```python
from build123d import *

# Parameters (mm, degrees)
ESQUISSE1_R                  = 53
ESQUISSE1_R_2                = 41
BOSS_EXTRU_1_DEPTH           = 3
ENL_V_MAT_EXTRU_1_DEPTH      = 76.013332148
ENL_V_MAT_EXTRU_1_DEPTH_BACK = 76.013332148
ENL_V_MAT_EXTRU_2_DEPTH      = 76.013332148
ENL_V_MAT_EXTRU_2_DEPTH_BACK = 76.013332148
CONG_1_R                     = 3
CONG_2_R                     = 2


with BuildPart() as part:
    # Esquisse1 → Boss.-Extru.1 (new body)
    with BuildSketch(Plane.XY):
        Circle(ESQUISSE1_R)
        Circle(ESQUISSE1_R_2, mode=Mode.SUBTRACT)
    extrude(amount=BOSS_EXTRU_1_DEPTH)

    # Esquisse2 → Enlèv. mat.-Extru.1 (cut, two sides: drawn at the far end of the back side and taken through both)
    with BuildSketch(Plane.XY.offset(3).offset(-ENL_V_MAT_EXTRU_1_DEPTH_BACK)):
        with BuildLine():
            Line((-18, 36.837480913), (-23.268292683, 47.619182643))
            ThreePointArc((-23.268292683, 47.619182643), (0, 53), (23.268292683, 47.619182643))
            Line((23.268292683, 47.619182643), (18, 36.837480913))
            ThreePointArc((18, 36.837480913), (0, 41), (-18, 36.837480913))
        make_face()
    extrude(amount=ENL_V_MAT_EXTRU_1_DEPTH + ENL_V_MAT_EXTRU_1_DEPTH_BACK, mode=Mode.SUBTRACT)

    # Esquisse3 → Enlèv. mat.-Extru.2 (cut, two sides: drawn at the far end of the back side and taken through both)
    with BuildSketch(Plane.XY.offset(3).offset(-ENL_V_MAT_EXTRU_2_DEPTH_BACK)):
        Polygon((26.024648968, -31.681503217), (31.681503217, -26.024648968), (35.924143904, -30.267289655), (30.267289655, -35.924143904), align=None)
        Polygon((-26.024648968, -31.681503217), (-30.267289655, -35.924143904), (-35.924143904, -30.267289655), (-31.681503217, -26.024648968), align=None)
        Polygon((-26.024648968, 31.681503217), (-31.681503217, 26.024648968), (-35.924143904, 30.267289655), (-30.267289655, 35.924143904), align=None)
        Polygon((26.024648968, 31.681503217), (30.267289655, 35.924143904), (35.924143904, 30.267289655), (31.681503217, 26.024648968), align=None)
    extrude(amount=ENL_V_MAT_EXTRU_2_DEPTH + ENL_V_MAT_EXTRU_2_DEPTH_BACK, mode=Mode.SUBTRACT)

    # Congé1
    cong_1_edges = [part.edges().sort_by_distance(p)[0] for p in [
        (-23.268292683, 47.619182643, 1.5),
        (23.268292683, 47.619182643, 1.5),
    ]]
    fillet(cong_1_edges, radius=CONG_1_R)

    # Congé2
    cong_2_edges = [part.edges().sort_by_distance(p)[0] for p in [
        (18, 36.837480913, 1.5),
        (-18, 36.837480913, 1.5),
        (30.267289655, 35.924143904, 1.5),
        (35.924143904, 30.267289655, 1.5),
        (-30.267289655, 35.924143904, 1.5),
        (-35.924143904, 30.267289655, 1.5),
        (-30.267289655, -35.924143904, 1.5),
        (-35.924143904, -30.267289655, 1.5),
        (35.924143904, -30.267289655, 1.5),
        (30.267289655, -35.924143904, 1.5),
    ]]
    fillet(cong_2_edges, radius=CONG_2_R)


solid = part.part
```
Work out the finished part from the listing and answer in its coordinate system (mm). A direction names the side the tool comes from. Coordinates: 2 decimals unless noted, no trailing zeros. Write each loop counter-clockwise with the first axis right and the second up, starting at its lowest first coordinate (ties: lowest second). Pieces come first, ordered by that corner, then holes.
Q1. Determine the mould class of faces 1 (the face through (41, 0, 1)), 2 (the face through (-1.949, -52.964, 1.479)), 3 (the face through (12, -40, 3)) for opening direction X: released by +X, released by -X, zero draft, split by the parting line, or undercut.
Q2. A cutting plane is placed at D-D, the plane x = 0. Give the vertices of the cut face in (y, z), then the cut area to 3 significant figures.
Q3. This flat-tipped pin is pushed along its axis until it touches: pin 1 Ø1.5 at (y, z) = (9, 2.5) entering from +X. Where does it stop, or does it pass through?
Q4. Find the intervals of material crossed by line 1 (Y direction, x = -19, z = 1.6); line 2 (X direction, y = 26, z = 2.35); line 3 (X direction, y = 25.5, z = 2.7), in increasing order.
Q5. A cutting plane is placed at A-A, the plane y = 0. Give the vertices of the cut face in (x, z).
Q6. Which of the six approach directions +Z, -Z, +X, -X, +Y, -Y give full straight-line access (tool end or side, diameter ignored) to faces 4 (the face through (20.406, 41.761, 1.479)), 5 (the face through (-41, 0, 1))?
Q7. A cutting plane is placed at C-C, the plane y = -21. Give the vertices of the cut face in (x, z).
Findings below:
1. face 1: undercut
1. face 2: split by the parting line
1. face 3: zero draft
2. outline: (-53, 0) - (-41, 0) - (-41, 3) - (-53, 3) - close
2. area: 36.0 mm2
3. pin 1: stops at x = 52.35
4. line 1: y = -49.48 to -36.33, 36.59 to 38.88
4. line 2: x = -46.18 to -31.7, 31.7 to 46.18
4. line 3: x = -46.46 to -32.11, 32.11 to 46.46
5. outline: (-53, 0) - (-41, 0) - (-41, 3) - (-53, 3) - close; (41, 0) - (53, 0) - (53, 3) - (41, 3) - close
6. face 4: +Z, -Z, +Y
6. face 5: +Z, -Z
7. outline: (-48.66, 0) - (-35.21, 0) - (-35.21, 3) - (-48.66, 3) - close; (35.21, 0) - (48.66, 0) - (48.66, 3) - (35.21, 3) - close
